from build123d import *

# Parameters (mm, degrees)
SKETCH_1_W          = 25
SKETCH_1_H          = 25
SKETCH_1_R          = 1.5
EXTRUDE_1_DEPTH     = 7
FILLET_1_R          = 2
SKETCH_2_R          = 11.5
CUT_EXTRUDE_1_DEPTH = 7


with BuildPart() as part:
    # 草图1 → 凸台-拉伸1 (new body)
    with BuildSketch(Plane(origin=(0, 0, 0), x_dir=(1, 0, 0), z_dir=(0, 1, 0))):
        Rectangle(SKETCH_1_W, SKETCH_1_H)
        with Locations(Location((-10, -10, 0), (0, 0, 270))):
            Circle(SKETCH_1_R, mode=Mode.SUBTRACT)
        with Locations(Location((10, -10, 0), (0, 0, 270))):
            Circle(SKETCH_1_R, mode=Mode.SUBTRACT)
        with Locations(Location((10, 10, 0), (0, 0, 270))):
            Circle(SKETCH_1_R, mode=Mode.SUBTRACT)
        with Locations(Location((-10, 10, 0), (0, 0, 270))):
            Circle(SKETCH_1_R, mode=Mode.SUBTRACT)
    extrude(amount=EXTRUDE_1_DEPTH)

    # 圆角1
    fillet_1_edges = [part.edges().sort_by_distance(p)[0] for p in [
        (12.5, 3.5, 12.5),
        (-12.5, 3.5, 12.5),
        (-12.5, 3.5, -12.5),
        (12.5, 3.5, -12.5),
    ]]
    fillet(fillet_1_edges, radius=FILLET_1_R)

    # 草图2 → 切除-拉伸1 (cut)
    with BuildSketch(Plane(origin=(0, 7, 0), x_dir=(1, 0, 0), z_dir=(0, 1, 0))):
        with Locations(Location((0, 0, 0), (0, 0, 270))):
            Circle(SKETCH_2_R)
    extrude(amount=-CUT_EXTRUDE_1_DEPTH, mode=Mode.SUBTRACT)


solid = part.part
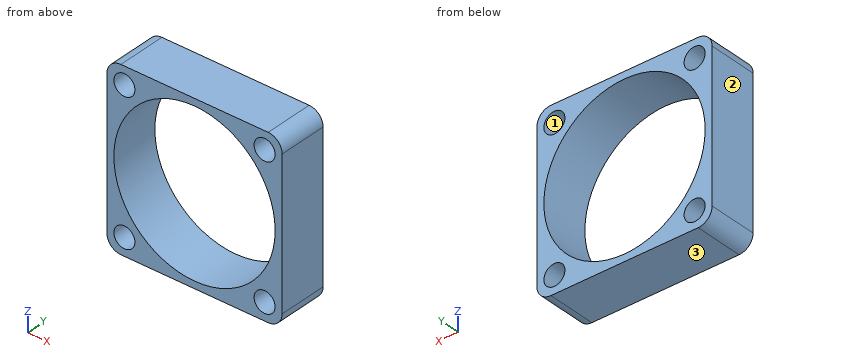
Can you work these out from the model? Positions are in its coordinate system, mm. Face numbers are marked on the shaded views. Give positions to 0.01 mm unless a question says otherwise; leave off trailing zeros. Write each loop counter-clockwise with the first axis right and the second up, starting at its lowest first coordinate (ties: lowest second). Pieces come first, ordered by that corner, then holes. Notation, with made-up numbers: (-18, 53) -> (6, 53) arc R9 cw to (6, 59) -> close; hole circle Ø4 at (49, 25.25). An arc over 180 degrees is marked (long way). Answer as a JSON object with one key per item and string values. Group by question number.
Item 1: Suppose I cut it at C-C (y = 4). Please give me the cut outline in (x, z), plus the area to 3 significant figures.
Item 2: Please list where these lines run through material, in increasing order: line 1 (X direction, y = 0.5, z = 9); line 2 (X direction, y = 2.25, z = 10); line 3 (Z direction, x = -10.5, y = 2). Write a range as [from, to].
Item 3: We'd pull the mould along X, two halves only. Please class the marked faces 1, 2 and 3: +X half, -X half, draft (parallel to the pull), parting line (faces both ways), or undercut.
Item 4: I'm going to push a flat-ended pin straight in: P1, Ø1.5, axis at x = -9.5, z = -7, coming from the -Y side. Where does the tip first touch, or does it pass through?
Item 5: Suppose I cut it at A-A (x = 6.5). Please give me the cut outline in (y, z).
Item 6: Suppose I cut it at D-D (x = -10). Please give me the cut outline in (y, z).
Item 7: Suppose I cut it at B-B (z = 0). Please give me the cut outline in (x, y), plus the area to 3 significant figures.
Findings:
{
 "1": {"outline": "(-12.5, -10.5) arc R2 ccw to (-10.5, -12.5) -> (10.5, -12.5) arc R2 ccw to (12.5, -10.5) -> (12.5, 10.5) arc R2 ccw to (10.5, 12.5) -> (-10.5, 12.5) arc R2 ccw to (-12.5, 10.5) -> close; hole circle Ø3 at (-10, -10); hole circle Ø23 at (0, 0); hole circle Ø3 at (-10, 10); hole circle Ø3 at (10, -10); hole circle Ø3 at (10, 10)", "area": "178 mm²"},
 "2": {"line 1": "x = [-12.5, -11.12], [-8.88, -7.16], [7.16, 8.88], [11.12, 12.5]", "line 2": "x = [-12.5, -11.5], [-8.5, -5.68], [5.68, 8.5], [11.5, 12.5]", "line 3": "z = [-12.5, -11.41], [-8.59, -4.69], [4.69, 8.59], [11.41, 12.5]"},
 "3": {"face 1": "undercut", "face 2": "-X half", "face 3": "draft"},
 "4": {"P1": "stops at y = 0"},
 "5": {"outline": "(0, -12.5) -> (7, -12.5) -> (7, -9.49) -> (0, -9.49) -> close; (0, 9.49) -> (7, 9.49) -> (7, 12.5) -> (0, 12.5) -> close"},
 "6": {"outline": "(0, -12.5) -> (7, -12.5) -> (7, -11.5) -> (0, -11.5) -> close; (0, -8.5) -> (7, -8.5) -> (7, -5.68) -> (0, -5.68) -> close; (0, 5.68) -> (7, 5.68) -> (7, 8.5) -> (0, 8.5) -> close; (0, 11.5) -> (7, 11.5) -> (7, 12.5) -> (0, 12.5) -> close"},
 "7": {"outline": "(-12.5, 0) -> (-11.5, 0) -> (-11.5, 7) -> (-12.5, 7) -> close; (11.5, 0) -> (12.5, 0) -> (12.5, 7) -> (11.5, 7) -> close", "area": "14.0 mm²"}
}
